Input: part model. Units: mm. Frame: model coordinates. Give positions to 0.01 mm unless a question says otherwise; leave off trailing zeros. Use CSV: the item, a comma, the result in double quotes. Start each with the question number.
from build123d import *

# Parameters (mm, degrees)
SKETCH_1_W          = 300
SKETCH_1_H          = 400
SKETCH_1_R          = 5
SKETCH_1_R_2        = 2
EXTRUDE_1_DEPTH     = 3
SKETCH_4_R          = 1.5
CUT_EXTRUDE_1_DEPTH = 251.017999352
SKETCH_5_R          = 1.5
CUT_EXTRUDE_2_DEPTH = 10
SKETCH_6_R          = 1.5
CUT_EXTRUDE_3_DEPTH = 251.017999352
SKETCH_7_R          = 15
CUT_EXTRUDE_4_DEPTH = 251.017999352
SKETCH_8_R          = 8
CUT_EXTRUDE_5_DEPTH = 10


with BuildPart() as part:
    # 草图1 → 凸台-拉伸1 (new body)
    with BuildSketch(Plane(origin=(0, 0, 0), x_dir=(1, 0, 0), z_dir=(0, 1, 0))):
        Rectangle(SKETCH_1_W, SKETCH_1_H)
        with Locations(Location((-137, 160, 0), (0, 0, 270))):
            Circle(SKETCH_1_R, mode=Mode.SUBTRACT)
        with Locations(Location((137, 160, 0), (0, 0, 270))):
            Circle(SKETCH_1_R, mode=Mode.SUBTRACT)
        with Locations(Location((137, -160, 0), (0, 0, 270))):
            Circle(SKETCH_1_R, mode=Mode.SUBTRACT)
        with Locations(Location((-137, -160, 0), (0, 0, 270))):
            Circle(SKETCH_1_R, mode=Mode.SUBTRACT)
        with Locations(Location((-144, 168, 0), (0, 0, 270))):
            Circle(SKETCH_1_R_2, mode=Mode.SUBTRACT)
        with Locations(Location((-130, 168, 0), (0, 0, 270))):
            Circle(SKETCH_1_R_2, mode=Mode.SUBTRACT)
        with Locations(Location((-130, 152, 0), (0, 0, 270))):
            Circle(SKETCH_1_R_2, mode=Mode.SUBTRACT)
        with Locations(Location((-144, 152, 0), (0, 0, 270))):
            Circle(SKETCH_1_R_2, mode=Mode.SUBTRACT)
        with Locations(Location((130, 152, 0), (0, 0, 90))):
            Circle(SKETCH_1_R_2, mode=Mode.SUBTRACT)
        with Locations(Location((144, 152, 0), (0, 0, 90))):
            Circle(SKETCH_1_R_2, mode=Mode.SUBTRACT)
        with Locations(Location((130, 168, 0), (0, 0, 90))):
            Circle(SKETCH_1_R_2, mode=Mode.SUBTRACT)
        with Locations(Location((144, 168, 0), (0, 0, 90))):
            Circle(SKETCH_1_R_2, mode=Mode.SUBTRACT)
        with Locations(Location((144, -152, 0), (0, 0, 270))):
            Circle(SKETCH_1_R_2, mode=Mode.SUBTRACT)
        with Locations(Location((130, -152, 0), (0, 0, 270))):
            Circle(SKETCH_1_R_2, mode=Mode.SUBTRACT)
        with Locations(Location((144, -168, 0), (0, 0, 270))):
            Circle(SKETCH_1_R_2, mode=Mode.SUBTRACT)
        with Locations(Location((130, -168, 0), (0, 0, 270))):
            Circle(SKETCH_1_R_2, mode=Mode.SUBTRACT)
        with Locations(Location((-144, -152, 0), (0, 0, 90))):
            Circle(SKETCH_1_R_2, mode=Mode.SUBTRACT)
        with Locations(Location((-130, -152, 0), (0, 0, 90))):
            Circle(SKETCH_1_R_2, mode=Mode.SUBTRACT)
        with Locations(Location((-130, -168, 0), (0, 0, 90))):
            Circle(SKETCH_1_R_2, mode=Mode.SUBTRACT)
        with Locations(Location((-144, -168, 0), (0, 0, 90))):
            Circle(SKETCH_1_R_2, mode=Mode.SUBTRACT)
    extrude(amount=EXTRUDE_1_DEPTH)

    # 草图4 → 切除-拉伸1 (cut, through all)
    with BuildSketch(Plane(origin=(0, 3, 0), x_dir=(1, 0, 0), z_dir=(0, 1, 0))):
        with Locations(Location((-142, -190, 0), (0, 0, 270))):
            Circle(SKETCH_4_R)
        with Locations(Location((142, -190, 0), (0, 0, 270))):
            Circle(SKETCH_4_R)
        with Locations(Location((142, 0, 0), (0, 0, 270))):
            Circle(SKETCH_4_R)
        with Locations(Location((-142, 0, 0), (0, 0, 270))):
            Circle(SKETCH_4_R)
        with Locations(Location((-142, 192, 0), (0, 0, 270))):
            Circle(SKETCH_4_R)
        with Locations(Location((142, 190, 0), (0, 0, 270))):
            Circle(SKETCH_4_R)
        with Locations(Location((0, 190, 0), (0, 0, 270))):
            Circle(SKETCH_4_R)
        with Locations(Location((0, -190, 0), (0, 0, 270))):
            Circle(SKETCH_4_R)
    extrude(amount=-CUT_EXTRUDE_1_DEPTH, mode=Mode.SUBTRACT)

    # 草图5 → 切除-拉伸2 (cut)
    with BuildSketch(Plane.XZ):
        with Locations(Location((-135, 120, 0), (0, 0, 270))):
            Circle(SKETCH_5_R)
        with Locations(Location((-90, 120, 0), (0, 0, 270))):
            Circle(SKETCH_5_R)
        with Locations(Location((-135, 75, 0), (0, 0, 270))):
            Circle(SKETCH_5_R)
        with Locations(Location((-90, 75, 0), (0, 0, 270))):
            Circle(SKETCH_5_R)
        with Locations(Location((90, 75, 0), (0, 0, 90))):
            Circle(SKETCH_5_R)
        with Locations(Location((135, 75, 0), (0, 0, 90))):
            Circle(SKETCH_5_R)
        with Locations(Location((90, 120, 0), (0, 0, 90))):
            Circle(SKETCH_5_R)
        with Locations(Location((135, 120, 0), (0, 0, 90))):
            Circle(SKETCH_5_R)
    extrude(amount=-CUT_EXTRUDE_2_DEPTH, mode=Mode.SUBTRACT)

    # 草图6 → 切除-拉伸3 (cut, through all)
    with BuildSketch(Plane.XZ):
        with Locations(Location((-35, 160, 0), (0, 0, 270))):
            Circle(SKETCH_6_R)
        with Locations(Location((35, 160, 0), (0, 0, 270))):
            Circle(SKETCH_6_R)
        with Locations(Location((-35, 90, 0), (0, 0, 270))):
            Circle(SKETCH_6_R)
        with Locations(Location((35, 90, 0), (0, 0, 270))):
            Circle(SKETCH_6_R)
    extrude(amount=-CUT_EXTRUDE_3_DEPTH, mode=Mode.SUBTRACT)

    # 草图7 → 切除-拉伸4 (cut, through all)
    with BuildSketch(Plane.XZ):
        with Locations(Location((0, 0, 0), (0, 0, 270))):
            Circle(SKETCH_7_R)
    extrude(amount=-CUT_EXTRUDE_4_DEPTH, mode=Mode.SUBTRACT)

    # 草图8 → 切除-拉伸5 (cut)
    with BuildSketch(Plane(origin=(0, 3, 0), x_dir=(1, 0, 0), z_dir=(0, 1, 0))):
        with Locations(Location((100, 185, 0), (0, 0, 270))):
            Circle(SKETCH_8_R)
    extrude(amount=-CUT_EXTRUDE_5_DEPTH, mode=Mode.SUBTRACT)


solid = part.part
Item 1: Material intervals for line 1 (X direction, y = 1.3, z = 190); line 2 (X direction, y = 2.1, z = 168); line 3 (Z direction, x = 90, y = 1.4), sorted ascending.
Item 2: First-contact query: pin 1 Ø3 at (x, z) = (144, 168) entering from -Y. Flat tip, straight axial feed; report the tip coordinate or a pass-through.
Item 3: Mould query, pull axis Z, two halves, no side actions, for faces 1 (the cylindrical face through (92.19, 1.52, -186.73)), 2 (the flat face through (-35, 3, -3)), 3 (the cylindrical face through (-137, 1, 155)). Classes: +Z half, -Z half, draft (parallel to the pull), parting line (faces both ways), or undercut.
Recorded:
1,line 1,"-150 to -143.5, -140.5 to -1.5, 1.5 to 140.5, 143.5 to 150"
1,line 2,"-150 to -146, -142 to -132, -128 to 128, 132 to 142, 146 to 150"
1,line 3,"-200 to 73.5, 76.5 to 118.5, 121.5 to 200"
2,pin 1,"through"
3,face 1,"undercut"
3,face 2,"draft"
3,face 3,"undercut"
